Geometry: final body of the model. Coordinates: model frame, mm. A direction names the side the tool comes from. Give positions to 0.01 mm unless a question says otherwise; leave off trailing zeros. Order: outer loops, then holes, each group sorted by start corner. A loop starts at its lowest first (then second) coordinate and runs counter-clockwise, first axis right, second up. Notation, with made-up numbers: (42, 31) -> (80, 31) arc R18 cw to (80, 52) -> close; hole circle Ø7 at (-29, 0). An arc over 180 degrees is marked (long way). One line per item, written item: value. Start each with the question number.
```python
from build123d import *

# Parameters (mm, degrees)
SKETCH_W         = 30
SKETCH_H         = 15.493133
REVOLUTION_ANGLE = 180


with BuildPart() as part:
    # Sketch → Revolution (revolve)
    with BuildSketch(Plane.XY):
        with Locations((20.143988, 12.253433)):
            Rectangle(SKETCH_W, SKETCH_H)
    revolve(axis=Axis((0, 0, 0), (1, 0, 0)), revolution_arc=REVOLUTION_ANGLE)

    # Sketch001 (on Face5 of Revolution) → Groove (revolve, cut)
    with BuildSketch(Plane(origin=(0, 0, 0), x_dir=(1, 0, 0), z_dir=(0, 0, -1))):
        with BuildLine():
            ThreePointArc((13.708482, 20.66012), (10.435215, 17.386853), (13.708482, 14.113586))
            Line((13.708482, 14.113586), (26.327395, 14.113586))
            ThreePointArc((26.327395, 14.113586), (29.600662, 17.386853), (26.327395, 20.66012))
            Line((13.708482, 20.66012), (26.327395, 20.66012))
        make_face()
    revolve(axis=Axis((0, 0, 0), (1, 0, 0)), mode=Mode.SUBTRACT)


solid = part.part
```
1. Cut plane B-B, the plane x = 19.25. Return loops of the section in (y, z), then the cut area to 3 significant figures.
2. Cut plane A-A, the plane y = 0. Return loops of the section in (x, z), then the cut area to 3 significant figures.
3. Cut plane C-C, the plane x = 9.5. Return loops of the section in (y, z), then the cut area to 3 significant figures.
4. Pin query (flat end, axial travel): P1, Ø10, axis at x = 10, z = 12.5, coming from the +Y side; P2, Ø2, axis at x = 15.5, y = 0, coming from the +Z side; P3, Ø4, axis at x = 23.5, z = 12, coming from the +Y side. Return the tip coordinate at first contact, or that it passes through.
5. Material intervals for L1, parallel to Z at x = 15.5, y = 0; L2, parallel to X at y = 6, z = 18; L3, parallel to X at y = 15.5, z = 11.5, sorted ascending. Write a range as [from, to].
6. Access query for faces 4 (the flat face through (35.144, 0, 10)), 5 (the cylindrical face through (20.11, 0.31, 14.11)). Directions: +Z, -Z, +X, -X, +Y, -Y. A direction counts if a zero-diameter tool reaches every point of the face in a straight line with its end or side. Return the directions, or none.
7. Draft query along Y for faces 1 (the cylindrical face through (20.354, 0.099, 4.506)), 2 (the cylindrical face through (32, 0, 20)), 3 (the flat face through (20, -11, 0)). Return one class per face: pulls with the +Y half, pulls with the -Y half, needs draft (parallel to the pull), parting line crosses it, or undercut.
Answers follow:
1. outline: (-14.11, 0) -> (-4.51, 0) arc R4.51 cw to (4.51, 0) -> (14.11, 0) arc R14.11 ccw to start
1. area: 281 mm²
2. outline: (5.14, 4.51) -> (35.14, 4.51) -> (35.14, 20) -> (28.3, 20) arc R3.27 cw to (26.33, 14.11) -> (13.71, 14.11) arc R3.27 cw to (11.74, 20) -> (5.14, 20) -> close
2. area: 359 mm²
3. outline: (-20, 0) -> (-4.51, 0) arc R4.51 cw to (4.51, 0) -> (20, 0) arc R20 ccw to start
3. area: 596 mm²
4. P1: stops at y = 18.54
4. P2: stops at z = 14.11
4. P3: stops at y = 9.96
5. L1: z = [4.51, 14.11]
5. L2: x = [5.14, 10.85], [29.19, 35.14]
5. L3: x = [5.14, 11.05], [28.98, 35.14]
6. face 4: +Z, -Z, +X, +Y, -Y
6. face 5: +Z
7. face 1: undercut
7. face 2: parting line crosses it
7. face 3: needs draft
